from build123d import *

# Parameters (mm, degrees)
F1_DEPTH      = 3.75
F1_DEPTH_BACK = 3.75
F2_W          = 12.5
F2_H          = 6.5
F3_DEPTH      = 0.501
F4_R          = 0.25
F5_DEPTH      = 4


with BuildPart() as f1:
    # F0 (on Top) → F1 (new body, two sides)
    with BuildSketch(Plane.XY) as f1_sk:
        with BuildLine():
            Line((6.25, 10), (-6.25, 10))
            Line((-6.25, 10), (-6.25, 0.5))
            Line((-6.25, 0.5), (-4.676025, 0.5))
            ThreePointArc((-4.676025, 0.5), (-3.81, 0), (-2.943975, 0.5))
            Line((-2.943975, 0.5), (2.943975, 0.5))
            ThreePointArc((2.943975, 0.5), (3.81, 0), (4.676025, 0.5))
            Line((4.676025, 0.5), (6.25, 0.5))
            Line((6.25, 0.5), (6.25, 10))
        make_face()
    extrude(amount=F1_DEPTH)
    extrude(f1_sk.sketch, amount=-F1_DEPTH_BACK)

    # F2 (on face) → F3 (cut, through all)
    with BuildSketch(Plane.XZ.offset(-0.5)):
        Rectangle(F2_W, F2_H)
    extrude(amount=F3_DEPTH, mode=Mode.SUBTRACT)

    # F4 (on face) → F5 (join)
    with BuildSketch(Plane.XZ.offset(-0.5)):
        with Locations((-5.18, 2.64)):
            Circle(F4_R)
        with Locations((-2.64, 2.64)):
            Circle(F4_R)
        with Locations((4.98, 2.64)):
            Circle(F4_R)
        with Locations((4.98, -2.825889)):
            Circle(F4_R)
        with Locations((-5.18, -2.825889)):
            Circle(F4_R)
        with Locations((-2.64, -2.825889)):
            Circle(F4_R)
    extrude(amount=F5_DEPTH)


solid = f1.part
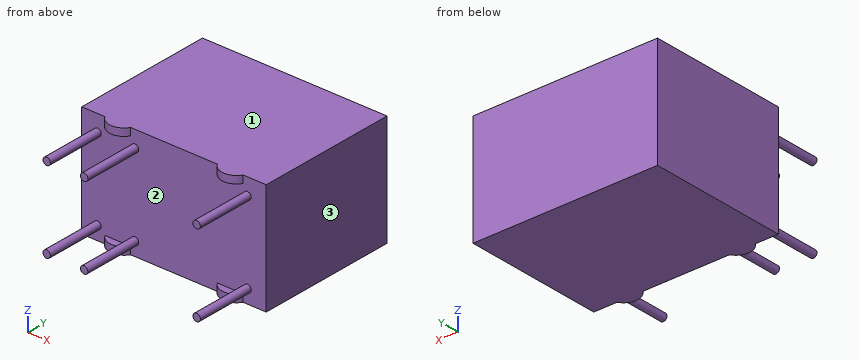
Geometry check sheet. Reference: the model listing, model coordinates, mm. Face numbers are marked on the shaded views. Coordinates: 2 decimals unless noted, no trailing zeros. Loops run counter-clockwise (first coordinate to the right, second up) from the corner with the lowest first, then second, coordinate; pieces in that order, holes last. Notation, with made-up numbers: (51, -16.75) - (66, -16.75) arc R7 cw to (66, -11.75) - close; hole circle Ø5 at (80, 61). An arc over 180 degrees is marked (long way). Use one line per item in the form item = value. Start each with the question number.
Item 1: Section check A-A, the plane x = 4.98. Enter the section's corners in (y, z).
Item 2: Thickness scan on probe 1 along Y at (x, z) = (-1, -1.5); probe 2 along Z at (x, y) = (-2.5, -3). Record the ranges inside material, lowest first.
Item 3: Gauge pin test, flat end, axial feed: pin 1 (1.5 mm diameter, centred on x = 4, z = -1, fed in from -Y). Record the tip position at first contact, or that the pin passes through.
Item 4: Section check B-B, the plane z = 2.64. Enter the section's corners in (x, y).
Item 5: Mould release check, pull along Z, two halves, no side actions. Record for the marked faces 1, 2 and 3: +Z half, -Z half, draft (parallel to the pull), parting line (faces both ways), or undercut.
Item 6: Section check D-D, the plane z = 0. Enter the section's corners in (x, y), and give its area (3 significant figures).
Item 7: Section check C-C, the plane y = -2. Enter the section's corners in (x, z).
Computed:
q1.outline = (-3.5, -3.08) - (0.5, -3.08) - (0.5, -3.75) - (10, -3.75) - (10, 3.75) - (0.5, 3.75) - (0.5, 2.89) - (-3.5, 2.89) - (-3.5, 2.39) - (0.5, 2.39) - (0.5, -2.58) - (-3.5, -2.58) - close
q2.probe_1 = 0.5 to 10
q2.probe_2 = -3.03 to -2.62, 2.43 to 2.85
q3.pin_1 = 0.5
q4.outline = (-6.25, 0.5) - (-5.43, 0.5) - (-5.43, -3.5) - (-4.93, -3.5) - (-4.93, 0.5) - (-2.89, 0.5) - (-2.89, -3.5) - (-2.39, -3.5) - (-2.39, 0.5) - (4.73, 0.5) - (4.73, -3.5) - (5.23, -3.5) - (5.23, 0.5) - (6.25, 0.5) - (6.25, 10) - (-6.25, 10) - close
q5.face_1 = +Z half
q5.face_2 = undercut
q5.face_3 = draft
q6.outline = (-6.25, 0.5) - (6.25, 0.5) - (6.25, 10) - (-6.25, 10) - close
q6.area = 119 mm2
q7.outline = circle Ø0.5 at (-5.18, -2.83); circle Ø0.5 at (-5.18, 2.64); circle Ø0.5 at (-2.64, -2.83); circle Ø0.5 at (-2.64, 2.64); circle Ø0.5 at (4.98, -2.83); circle Ø0.5 at (4.98, 2.64)
